```python
from build123d import *

# Parameters (mm, degrees)
SKETCH1_W           = 14.5
SKETCH1_H           = 38
SKETCH1_W_2         = 10.5
SKETCH1_H_2         = 2.2
BOSS_EXTRUDE1_DEPTH = 0.9
SKETCH2_W           = 14.5
SKETCH2_H           = 8.05
BOSS_EXTRUDE2_DEPTH = 6
DRAFT1_ANGLE        = 2
SKETCH2_3_W         = 14.5
SKETCH2_3_H         = 6.2
SKETCH2_3_W_2       = 10.5
SKETCH2_3_H_2       = 2.2
BOSS_EXTRUDE3_DEPTH = 3
CHAMFER1_SIZE       = 5
CHAMFER1_SIZE2      = 6.399708161
FILLET2_R           = 1
FILLET3_R           = 1
FILLET4_R           = 5
FILLET5_R           = 0.8


with BuildPart() as part:
    # Sketch1 → Boss-Extrude1 (new body)
    with BuildSketch(Plane.XY):
        with Locations((0, 16)):
            Rectangle(SKETCH1_W, SKETCH1_H)
        with Locations((0, 1.1)):
            Rectangle(SKETCH1_W_2, SKETCH1_H_2, mode=Mode.SUBTRACT)
    extrude(amount=BOSS_EXTRUDE1_DEPTH)

    # Sketch2 → Boss-Extrude2 (add)
    with BuildSketch(Plane.XY.offset(0.9)):
        with Locations((0, 30.975)):
            Rectangle(SKETCH2_W, SKETCH2_H)
    extrude(amount=BOSS_EXTRUDE2_DEPTH)

    # Draft1
    draft1_faces = [part.faces().sort_by_distance(p)[0] for p in [
        (0, 26.95, 3.9),
    ]]
    draft(draft1_faces, Plane.XY.offset(0.9), DRAFT1_ANGLE)

    # Sketch2<3> → Boss-Extrude3 (add)
    with BuildSketch(Plane.XY.offset(0.9)):
        with Locations((0, 1.1)):
            Rectangle(SKETCH2_3_W, SKETCH2_3_H)
        with Locations((0, 1.1)):
            Rectangle(SKETCH2_3_W_2, SKETCH2_3_H_2, mode=Mode.SUBTRACT)
    extrude(amount=BOSS_EXTRUDE3_DEPTH)

    # Chamfer1
    chamfer1_edges = [part.edges().sort_by_distance(p)[0] for p in [
        (0, 35, 6.9),
    ]]
    chamfer1_side = [part.faces().sort_by_distance(p)[0] for p in [
        (0, 35, 3.45),
    ]]
    chamfer(chamfer1_edges, length=CHAMFER1_SIZE, length2=CHAMFER1_SIZE2, reference=chamfer1_side[0])

    # Fillet2
    fillet2_edges = [part.edges().sort_by_distance(p)[0] for p in [
        (0, 27.159524617, 6.9),
    ]]
    fillet(fillet2_edges, radius=FILLET2_R)

    # Fillet3
    fillet3_edges = [part.edges().sort_by_distance(p)[0] for p in [
        (0, 26.95, 0.9),
        (0, 4.2, 0.9),
    ]]
    fillet(fillet3_edges, radius=FILLET3_R)

    # Fillet4
    fillet4_edges = [part.edges().sort_by_distance(p)[0] for p in [
        (-7.25, 35, 0.95),
        (7.25, 35, 0.95),
    ]]
    fillet(fillet4_edges, radius=FILLET4_R)

    # Fillet5
    fillet5_edges = [part.edges().sort_by_distance(p)[0] for p in [
        (7.25, -2, 2.4),
        (-7.25, -2, 2.4),
        (0, 0, 3.9),
        (-5.25, 1.1, 3.9),
        (0, 2.2, 3.9),
        (5.25, 1.1, 3.9),
        (7.25, -3, 0.45),
        (-7.25, -3, 0.45),
    ]]
    fillet(fillet5_edges, radius=FILLET5_R)


solid = part.part
```
Source: CAD feature listing. Evaluate the final solid. Frame: model axes, mm. A direction names the side the tool comes from. Round coordinates to 2 decimals unless told otherwise and drop trailing zeros. Write each loop counter-clockwise with the first axis right and the second up, starting at its lowest first coordinate (ties: lowest second). Pieces come first, ordered by that corner, then holes. Notation, with made-up numbers: M -37,19.25 L -28,19.25 A16 ccw -28,23.25 Z; hole C 27.5,-15.75 d6. An arc over 180 degrees is marked long. Answer as a JSON object with one key per item and string values. Group by question number.
(1) Ray query, line 1 (Y direction, x = -5, z = 2); line 2 (Y direction, x = 0.5, z = 1); line 3 (X direction, y = 1, z = 1.5). Return the intervals inside material, ascending. Write a range as [from, to].
(2) First-contact query: pin 1 (1.9 mm diameter, centred on x = -1, y = 1, fed in from +Z); pin 2 (3 mm diameter, centred on x = -3.5, y = 3, fed in from +Z); pin 3 (3 mm diameter, centred on x = 5, z = 2.5, fed in from -Y); pin 4 (0.6 mm diameter, centred on x = -2.5, z = 3.5, fed in from +Y). Flat tips, straight axial feed; report the tip coordinate or a pass-through.
(3) Reachability of faces 1 (the cylindrical face through (0.08, -0.24, 3.67)), 2 (the cylindrical face through (0.1, 26.7, 1.2)), 3 (the flat face through (-5.25, 1, 2)) from +Z, -Z, +X, -X, +Y, -Y: full face, straight path, thin tool, end or side. Return the list, or none.
(4) Section query B-B on z = 2.75. Output: boundary loops of the cut face in (x, y), then the cut area to 3 significant figures.
(5) Section query A-A on x = 0. Output: boundary loops of the cut face in (y, z), then the cut area to 3 significant figures.
(6) Section query C-C on y = 24.5. Output: boundary loops of the cut face in (x, z), then the cut area to 4 significant figures.
(7) Mould query, pull axis X, two halves, no side actions, for faces 4 (the flat face through (7.25, 13.8, 0.4)), 5 (the flat face through (0, 4.2, 3)), 6 (the cylindrical face through (5.6, 1.13, 3.76)). Classes: +X half, -X half, draft (parallel to the pull), parting line (faces both ways), or undercut.
(8) Section query D-D on x = -4.75. Output: boundary loops of the cut face in (y, z).
Computed values:
{
 "1": {"line 1": "[-2, 0], [2.2, 4.2], [26.99, 34.18]", "line 2": "[-2, 0], [2.2, 4.76], [26.42, 35]", "line 3": "[-7.25, -5.25], [5.25, 7.25]"},
 "2": {"pin 1": "through", "pin 2": "z = 3.9", "pin 3": "y = -2", "pin 4": "y = 33.34"},
 "3": {"face 1": "+Z", "face 2": "+Z, +X, -X", "face 3": "+Z, -Z"},
 "4": {"outline": "M -7.25,-1.2 A0.8 ccw -6.45,-2 L 6.45,-2 A0.8 ccw 7.25,-1.2 L 7.25,4.2 L -7.25,4.2 Z; M -7.25,27.01 L 7.25,27.01 L 7.25,30 A5 ccw 5.36,33.91 L -5.36,33.91 A5 ccw -7.25,30 Z; hole M -5.25,0 L 5.25,0 L 5.25,2.2 L -5.25,2.2 Z", "area": "162 mm^2"},
 "5": {"outline": "M -3,0 L 0,0 L 0,3.1 A0.8 ccw -0.8,3.9 L -2,3.9 L -2,0.9 L -3,0.9 Z; M 2.2,0 L 35,0 L 35,1.9 L 28.6,6.9 L 28.13,6.9 A1 ccw 27.13,5.93 L 26.98,1.87 A1 cw 25.98,0.9 L 5.2,0.9 A1 cw 4.2,1.9 L 4.2,3.9 L 3,3.9 A0.8 ccw 2.2,3.1 Z", "area": "75.8 mm^2"},
 "6": {"outline": "M -7.25,0 L 7.25,0 L 7.25,0.9 L -7.25,0.9 Z", "area": "13.05 mm^2"},
 "7": {"face 4": "+X half", "face 5": "draft", "face 6": "undercut"},
 "8": {"outline": "M -3,0 L 0,0 L 0,3.1 A0.8 ccw -0.8,3.9 L -2,3.9 L -2,0.9 L -3,0.9 Z; M 2.2,0 L 34.33,0 L 34.33,2.42 L 28.6,6.9 L 28.13,6.9 A1 ccw 27.13,5.93 L 26.98,1.87 A1 cw 25.98,0.9 L 5.2,0.9 A1 cw 4.2,1.9 L 4.2,3.9 L 3,3.9 A0.8 ccw 2.2,3.1 Z"}
}
